Design review of the part built by this model. Coordinates are the model's own, in mm. A direction names the side the tool comes from. Coordinates: 2 decimals unless noted, no trailing zeros. Loops run counter-clockwise (first coordinate to the right, second up) from the corner with the lowest first, then second, coordinate; pieces in that order, holes last. Notation, with made-up numbers: (-19, -38) -> (-13, -38) arc R18 ccw to (-13, -27) -> close; hole circle Ø2 at (19, -36.75). An arc over 180 degrees is marked (long way). One line per item, written item: value. Start each with the question number.
1. Draft analysis for pull direction X (two halves, no side actions). For faces 4 (the cylindrical face through (7.097, 5.67, 6.15)), 5 (the flat face through (3, 0, 3)), state which applies: pulls with the +X half, pulls with the -X half, needs draft (parallel to the pull), parting line crosses it, or undercut.
2. For probe 1 along Z at (x, y) = (4, 3.25); probe 2 along Z at (x, y) = (0, 7.5); probe 3 along Z at (x, y) = (5.5, 2.5), list the stretches that pass through material, from the lowest coordinate up.
3. Machinability: for faces 1 (the cylindrical face through (-11.4, 13, 14.2)), 2 (the cylindrical face through (2.98, 13.274, -3.563)), 3 (the flat face through (0, 11, -13)), which of the approach directions +Z, -Z, +X, -X, +Y, -Y give a long, thin tool a straight path to every point of the face, cutting with its end or side? Answer none if there is none.
4. Insertion check: pin 1 (3 mm diameter, centred on x = 4, z = 4.5, fed in from +Y); pin 2 (4.5 mm diameter, centred on x = -6.31, z = -15.24, fed in from -Y); pin 3 (5.5 mm diameter, centred on x = -5.48, z = -5.48, fed in from +Y); pin 4 (8 mm diameter, centred on x = 12.5, y = 12, fed in from -Z). Each pin has a flat end and moves straight along its axis. Give the tip position at first contact, or say it passes through.
5. Add section B-B on x = 6.5. Give the number of separate pieces and of enclosed holes in the cut face, plus the area to 3 significant figures.
6. Add section A-A on x = 0. Write out the cut boundary in (y, z), plus the area to 3 significant figures.
```python
from build123d import *

# Parameters (mm, degrees)
SKETCH1_R      = 20.05
SKETCH1_R_2    = 3.25
SKETCH1_R_3    = 1.75
EXTRUDE1_DEPTH = 15
SKETCH7_R      = 3.15
EXTRUDE4_DEPTH = 3.5
SKETCH8_R      = 20.05
SKETCH8_R_2    = 12.5
EXTRUDE5_DEPTH = 11
FILLET_1_R     = 0.5


with BuildPart() as part:
    # Sketch1 → Extrude1 (new body)
    with BuildSketch(Plane(origin=(0, 0, 0), x_dir=(1, 0, 0), z_dir=(0, 1, 0))):
        Circle(SKETCH1_R)
        Circle(SKETCH1_R_2, mode=Mode.SUBTRACT)
        with Locations((5.480077554, 5.480077554)):
            Circle(SKETCH1_R_3, mode=Mode.SUBTRACT)
        with Locations((5.480077554, -5.480077554)):
            Circle(SKETCH1_R_3, mode=Mode.SUBTRACT)
        with Locations((-5.480077554, -5.480077554)):
            Circle(SKETCH1_R_3, mode=Mode.SUBTRACT)
        with Locations((-5.480077554, 5.480077554)):
            Circle(SKETCH1_R_3, mode=Mode.SUBTRACT)
        with Locations((-10.044563579, -13.090330115)):
            Circle(SKETCH1_R_3, mode=Mode.SUBTRACT)
        with Locations((-6.314276634, 15.244012286)):
            Circle(SKETCH1_R_3, mode=Mode.SUBTRACT)
        with Locations((16.358840213, -2.153682172)):
            Circle(SKETCH1_R_3, mode=Mode.SUBTRACT)
    extrude(amount=EXTRUDE1_DEPTH)

    # Sketch7 → Extrude4 (cut)
    with BuildSketch(Plane(origin=(0, 15, 0), x_dir=(1, 0, 0), z_dir=(0, 1, 0))):
        with Locations((-5.480077554, 5.480077554)):
            Circle(SKETCH7_R)
        with Locations((5.480077554, 5.480077554)):
            Circle(SKETCH7_R)
        with Locations((5.480077554, -5.480077554)):
            Circle(SKETCH7_R)
        with Locations((-5.480077554, -5.480077554)):
            Circle(SKETCH7_R)
    extrude(amount=-EXTRUDE4_DEPTH, mode=Mode.SUBTRACT)

    # Sketch8 → Extrude5 (cut)
    with BuildSketch(Plane.XZ):
        Circle(SKETCH8_R)
        Circle(SKETCH8_R_2, mode=Mode.SUBTRACT)
    extrude(amount=-EXTRUDE5_DEPTH, mode=Mode.SUBTRACT)

    # 圓角1
    fillet_1_edges = [part.edges().sort_by_distance(p)[0] for p in [
        (-20.05, 15, 0),
    ]]
    fillet(fillet_1_edges, radius=FILLET_1_R)


solid = part.part
```
Worked answers:
1. face 4: undercut
1. face 5: needs draft
2. probe 1: z = -11.84 to -6.41, -4.55 to 4.55, 6.41 to 11.84
2. probe 2: z = -12.5 to -3.25, 3.25 to 12.5
2. probe 3: z = -11.22 to -7.23, -3.73 to 3.73, 7.23 to 11.22
3. face 1: +Y, -Y
3. face 2: +Y
3. face 3: -Y
4. pin 1: stops at y = 15
4. pin 2: stops at y = 11
4. pin 3: stops at y = 11.5
4. pin 4: stops at z = -18.16
5. separate pieces: 3
5. enclosed holes: 0
5. area: 279 mm²
6. outline: (0, -12.5) -> (11, -12.5) -> (11, -20.05) -> (14.5, -20.05) arc R0.5 ccw to (15, -19.55) -> (15, -3.25) -> (0, -3.25) -> close; (0, 3.25) -> (15, 3.25) -> (15, 19.55) arc R0.5 ccw to (14.5, 20.05) -> (11, 20.05) -> (11, 12.5) -> (0, 12.5) -> close
6. area: 338 mm²
